Autodesk Inventor part; units mm, degrees
ref_plane "YZ Plane" through (0, 0, 0) normal (1, 0, 0) x (0, 1, 0)
ref_plane "XZ Plane" through (0, 0, 0) normal (0, 1, 0) x (-1, 0, 0)
ref_plane "XY Plane" through (0, 0, 0) normal (0, 0, 1) x (1, 0, 0)
sketch "Sketch1" plane through (0, 0, 0) normal (0, 0, 1) x (1, 0, 0)
  line L0 (-22.0527, 33.1775) -> (28.7473, 33.1775)
  line L1 (28.7473, 33.1775) -> (28.7473, -652.6225)
  line L2 (28.7473, -652.6225) -> (-22.0527, -652.6225)
  line L3 (-22.0527, -652.6225) -> (-22.0527, 33.1775)
  point P0 (0, 0)
  dimension "d0" = 50.8
  dimension "d1" = 685.8
extrude "Extrusion1" add sketch "Sketch1" along normal blind 25.4
sketch "Sketch2" plane through (-22.0527, 33.1775, 0) normal (0, 1, 0) x (1, 0, 0)
  line L0 (0, 0) -> (0, -25.4)
  line L1 (0, 0) -> (50.8, 0)
  line L2 (50.8, 0) -> (50.8, -25.4)
  line L3 (50.8, -25.4) -> (0, -25.4)
  line L4 (6.35, -19.05) -> (6.35, -6.35)
  line L5 (6.35, -6.35) -> (44.45, -6.35)
  line L6 (44.45, -6.35) -> (44.45, -19.05)
  line L7 (44.45, -19.05) -> (6.35, -19.05)
  point P0 (22.0527, 0)
  dimension "d4" = 6.35
extrude "Extrusion2" cut sketch "Sketch2" against normal through all contours L4 L5 L6 L7
sketch "Sketch3" plane through (-22.0527, -652.6225, 0) normal (-1, 0, 0) x (0, 0, 1)
  line L0 (0, 685.8) -> (25.4, 685.8)
  line L1 (12.7, 685.8) -> (12.7, 0) construction
  line L2 (6.35, 0) -> (19.05, 0)
  circle A0 centre (12.7, 660.4) radius 3.175
  point P0 (0, 652.6225)
  dimension "d7" = 6.35
  dimension "d8" = 25.4
extrude "Extrusion3" cut sketch "Sketch3" against normal through all
pattern_linear "Rectangular Pattern1" count 26 spacing 25.4 along (0, -1, 0) of "Extrusion3"
properties part number "2AM-17-02-Back Frame" material "Aluminum 6061"
Work out the finished part from the listing and answer in its coordinate system (mm). A direction names the side the tool comes from. Coordinates: 2 decimals unless noted, no trailing zeros. Write each loop counter-clockwise with the first axis right and the second up, starting at its lowest first coordinate (ties: lowest second). Pieces come first, ordered by that corner, then holes.
Q1. A cutting plane is placed at A-A, the plane x = -5.5. Give the vertices of the cut face in (y, z).
Q2. Which of the six approach directions +Z, -Z, +X, -X, +Y, -Y give full straight-line access (tool end or side, diameter ignored) to faces 5 (the face through (3, -305, 0)), 6 (the face through (22.397, -305, 13))?
Q3. Determine the mould class of faces 1 (the face through (3, -305, 25.4)), 2 (the face through (28.747, -305, 13)), 3 (the face through (-22.053, -315, 13)), 4 (the face through (4, -305, 19.05)) for opening direction X: released by +X, released by -X, zero draft, split by the parting line, or undercut.
Q4. Find the intervals of material crossed by line 1 (Z direction, x = 22, y = -193); line 2 (X direction, y = -253.5, z = 18); line 3 (Z direction, x = -18, y = -273), in increasing order.
Findings below:
1. outline: (-652.62, 0) - (33.18, 0) - (33.18, 6.35) - (-652.62, 6.35) - close; (-652.62, 19.05) - (33.18, 19.05) - (33.18, 25.4) - (-652.62, 25.4) - close
2. face 5: -Z, +X, -X, +Y, -Y
2. face 6: +Y, -Y
3. face 1: zero draft
3. face 2: released by +X
3. face 3: released by -X
3. face 4: undercut
4. line 1: z = 0 to 6.35, 19.05 to 25.4
4. line 2: x = -22.05 to -15.7, 22.4 to 28.75
4. line 3: z = 0 to 9.84, 15.56 to 25.4
